from build123d import *

# Parameters (mm, degrees)
BOSS_EXTRUDE1_DEPTH = 3
SKETCH2_W           = 90
SKETCH2_H           = 44
CUT_EXTRUDE1_DEPTH  = 10
FILLET1_R           = 10
CHAMFER1_SIZE       = 15
SKETCH3_W           = 85
SKETCH3_H           = 1.6
CUT_EXTRUDE2_DEPTH  = 10
SKETCH5_W           = 3
SKETCH5_H           = 13
SKETCH5_H_2         = 8.82
SKETCH5_W_2         = 18
SKETCH5_H_3         = 3
SKETCH5_H_4         = 22.31
CUT_EXTRUDE3_DEPTH  = 10
CUT_EXTRUDE4_DEPTH  = 10
SKETCH7_R           = 10.631131443
SKETCH7_R_2         = 8.661974079
SKETCH7_R_3         = 5.563912072
SKETCH7_R_4         = 5.743787148
SKETCH7_R_5         = 6.57513677
SKETCH7_R_6         = 8.998042507
SKETCH7_R_7         = 11.788086797
SKETCH7_R_8         = 9.954868747
SKETCH7_R_9         = 6.082926802
SKETCH7_R_10        = 4.464279257
SKETCH7_R_11        = 4.037680116
SKETCH7_R_12        = 3.945902669
CUT_EXTRUDE5_DEPTH  = 10


with BuildPart() as part:
    # Sketch1 → Boss-Extrude1 (new body)
    with BuildSketch(Plane.XY):
        with BuildLine():
            Line((-45, 96.5), (45, 96.5))
            ThreePointArc((45, 96.5), (66.213203436, 87.713203436), (75, 66.5))
            Line((75, 66.5), (75, -56.5))
            ThreePointArc((75, -56.5), (63.284271247, -84.784271247), (35, -96.5))
            Line((35, -96.5), (0.5, -96.5))
            Line((0.5, -96.5), (-0.5, -96.5))
            Line((-0.5, -96.5), (-35, -96.5))
            ThreePointArc((-35, -96.5), (-63.284271247, -84.784271247), (-75, -56.5))
            Line((-75, -56.5), (-75, 66.5))
            ThreePointArc((-75, 66.5), (-66.213203436, 87.713203436), (-45, 96.5))
        make_face()
    extrude(amount=BOSS_EXTRUDE1_DEPTH)

    # Sketch2 → Cut-Extrude1 (cut)
    with BuildSketch(Plane.XY.offset(3)):
        with Locations((0, -34.5)):
            Rectangle(SKETCH2_W, SKETCH2_H)
    extrude(amount=-CUT_EXTRUDE1_DEPTH, mode=Mode.SUBTRACT)

    # Fillet1
    fillet1_edges = [part.edges().sort_by_distance(p)[0] for p in [
        (45, -56.5, 1.5),
        (-45, -56.5, 1.5),
    ]]
    fillet(fillet1_edges, radius=FILLET1_R)

    # Chamfer1
    chamfer1_edges = [part.edges().sort_by_distance(p)[0] for p in [
        (45, -12.5, 1.5),
        (-45, -12.5, 1.5),
    ]]
    chamfer(chamfer1_edges, length=CHAMFER1_SIZE)

    # Sketch3 → Cut-Extrude2 (cut)
    with BuildSketch(Plane(origin=(0, 0, 0), x_dir=(-1, 0, 0), z_dir=(0, 0, -1))):
        with Locations((0, -13.3)):
            Rectangle(SKETCH3_W, SKETCH3_H)
    extrude(amount=-CUT_EXTRUDE2_DEPTH, mode=Mode.SUBTRACT)

    # Sketch5 → Cut-Extrude3 (cut)
    with BuildSketch(Plane(origin=(0, 0, 0), x_dir=(-1, 0, 0), z_dir=(0, 0, -1))):
        with Locations((-73.5, 60)):
            Rectangle(SKETCH5_W, SKETCH5_H)
        with Locations((-40.5, 85.09)):
            Rectangle(SKETCH5_W, SKETCH5_H_2)
        with Locations((73.5, 60)):
            Rectangle(SKETCH5_W, SKETCH5_H)
        with Locations((40.5, 85.09)):
            Rectangle(SKETCH5_W, SKETCH5_H_2)
        with Locations((-49, -62.69)):
            Rectangle(SKETCH5_W_2, SKETCH5_H_3)
        with Locations((49, -62.69)):
            Rectangle(SKETCH5_W_2, SKETCH5_H_3)
        with Locations((28.5, -85.345)):
            Rectangle(SKETCH5_W, SKETCH5_H_4)
        with Locations((-28.5, -85.345)):
            Rectangle(SKETCH5_W, SKETCH5_H_4)
    extrude(amount=-CUT_EXTRUDE3_DEPTH, mode=Mode.SUBTRACT)

    # Sketch6 → Cut-Extrude4 (cut)
    with BuildSketch(Plane(origin=(0, 0, 0), x_dir=(-1, 0, 0), z_dir=(0, 0, -1))):
        with BuildLine():
            Line((-24.212655847, 72.63796754), (24.212655847, 72.63796754))
            ThreePointArc((24.212655847, 72.63796754), (58.665446775, 38.185176612), (24.212655847, 3.732385684))
            Line((24.212655847, 3.732385684), (-24.212655847, 3.732385684))
            ThreePointArc((-24.212655847, 3.732385684), (-58.665446775, 38.185176612), (-24.212655847, 72.63796754))
        make_face()
    extrude(amount=-CUT_EXTRUDE4_DEPTH, mode=Mode.SUBTRACT)

    # Sketch7 → Cut-Extrude5 (cut)
    with BuildSketch(Plane(origin=(0, 0, 0), x_dir=(-1, 0, 0), z_dir=(0, 0, -1))):
        with Locations((-56.155531371, 77.040268603)):
            Circle(SKETCH7_R)
        with Locations((-26.105041506, 84.696444365)):
            Circle(SKETCH7_R_2)
        with Locations((-63.23749395, 58.091233593)):
            Circle(SKETCH7_R_3)
        with Locations((-66.021045237, 42.587477675)):
            Circle(SKETCH7_R_4)
        with Locations((-66.021045237, 25.361082211)):
            Circle(SKETCH7_R_5)
        with Locations((-58.260979705, 4.306598866)):
            Circle(SKETCH7_R_6)
        with Locations((-60.749236828, -19.427545996)):
            Circle(SKETCH7_R_7)
        with Locations((-59.983619252, -46.60696995)):
            Circle(SKETCH7_R_8)
        with Locations((-8.495837254, 84.696444365)):
            Circle(SKETCH7_R_9)
        with Locations((-39.120540301, -6.220642806)):
            Circle(SKETCH7_R_10)
        with Locations((-26.105041506, -6.220642806)):
            Circle(SKETCH7_R_11)
        with Locations((-13.855160287, -6.220642806)):
            Circle(SKETCH7_R_12)
        with Locations((13.855160287, -6.220642806)):
            Circle(SKETCH7_R_12)
        with Locations((26.105041506, -6.220642806)):
            Circle(SKETCH7_R_11)
        with Locations((39.120540301, -6.220642806)):
            Circle(SKETCH7_R_10)
        with Locations((8.495837254, 84.696444365)):
            Circle(SKETCH7_R_9)
        with Locations((59.983619252, -46.60696995)):
            Circle(SKETCH7_R_8)
        with Locations((60.749236828, -19.427545996)):
            Circle(SKETCH7_R_7)
        with Locations((58.260979705, 4.306598866)):
            Circle(SKETCH7_R_6)
        with Locations((66.021045237, 25.361082211)):
            Circle(SKETCH7_R_5)
        with Locations((66.021045237, 42.587477675)):
            Circle(SKETCH7_R_4)
        with Locations((63.23749395, 58.091233593)):
            Circle(SKETCH7_R_3)
        with Locations((26.105041506, 84.696444365)):
            Circle(SKETCH7_R_2)
        with Locations((56.155531371, 77.040268603)):
            Circle(SKETCH7_R)
    extrude(amount=-CUT_EXTRUDE5_DEPTH, mode=Mode.SUBTRACT)


solid = part.part
Source: CAD feature listing. Evaluate the final solid. Frame: model axes, mm. A direction names the side the tool comes from. Coordinates: 2 decimals unless noted, no trailing zeros. Loops run counter-clockwise (first coordinate to the right, second up) from the corner with the lowest first, then second, coordinate; pieces in that order, holes last. Notation, with made-up numbers: (-40, -13.75) - (1, -13.75) arc R18 ccw to (1, 3.25) - close; hole circle Ø1 at (20, 64.25). An arc over 180 degrees is marked (long way). One line per item, written item: value. Start each with the question number.
1. Section C-C (x = 4.5). Return the cut outline in (y, z), and give its area (3 significant figures).
2. Section A-A (x = -53.5). Return the cut outline in (y, z), and give its area (3 significant figures).
3. Section D-D (z = 1.45). State how many separate pieces and enclosed holes the cut face has, and give its area (3 significant figures).
4. Mould query, pull axis X, two halves, no side actions, for faces 1 (the cylindrical face through (-66.573, 0.86, 1.479)), 2 (the cylindrical face through (-62.972, -85.094, 1.479)), 3 (the cylindrical face through (65.979, 87.945, 1.479)). Classes: pulls with the +X half, pulls with the -X half, needs draft (parallel to the pull), parting line crosses it, or undercut.
5. Contact query for flat-ended pins moving along their axis: P1, Ø13, axis at x = 56.16, y = 77.04, coming from the -Z side; P2, Ø0.9, axis at y = -63, z = 1, coming from the -X side; P3, Ø1.5, axis at y = 58, z = 2, coming from the -X side; P4, Ø1, axis at y = 68.5, z = 2, coming from the +X side. Output: stop coordinate, or through.
6. Set-up query: faces 4 (the flat face through (-38.4, -20.9, 1.5)), 5 (the cylindrical face through (63.594, -84.472, 1.479)). Return all of +Z, -Z, +X, -X, +Y, -Y with unobstructed straight access to the full face (end or side cutting, diameter ignored); none if empty.
7. Section B-B (y = -83). Return the cut outline in (x, z).
8. Ray query, L1, parallel to X at y = -47, z = 2.65; L2, parallel to Y at x = -68, z = 0.7; L3, parallel to X at y = 68.5, z = 1.2. Return the intervals inside material, ascending.
Verdict:
1. outline: (-96.5, 0) - (-56.5, 0) - (-56.5, 3) - (-96.5, 3) - close; (-12.5, 0) - (3.73, 0) - (3.73, 3) - (-12.5, 3) - close; (72.64, 0) - (80.11, 0) - (80.11, 3) - (72.64, 3) - close; (89.28, 0) - (96.5, 0) - (96.5, 3) - (89.28, 3) - close
1. area: 213 mm2
2. outline: (-91.96, 0) - (-64.19, 0) - (-64.19, 3) - (-91.96, 3) - close; (-61.19, 0) - (-54.16, 0) - (-54.16, 3) - (-61.19, 3) - close; (-39.05, 0) - (-28.72, 0) - (-28.72, 3) - (-39.05, 3) - close; (-10.13, 0) - (-3.33, 0) - (-3.33, 3) - (-10.13, 3) - close; (11.94, 0) - (20.04, 0) - (20.04, 3) - (11.94, 3) - close; (56.33, 0) - (66.75, 0) - (66.75, 3) - (56.33, 3) - close; (87.33, 0) - (95.27, 0) - (95.27, 3) - (87.33, 3) - close
2. area: 235 mm2
3. separate pieces: 1
3. enclosed holes: 30
3. area: 12,300 mm2
4. face 1: undercut
4. face 2: pulls with the -X half
4. face 3: pulls with the +X half
5. P1: passes through
5. P2: stops at x = -74.54
5. P3: stops at x = -72
5. P4: stops at x = 74.96
6. face 4: +Z, -Z
6. face 5: +Z, -Z, +X, -Y
7. outline: (-64.96, 0) - (-30, 0) - (-30, 3) - (-64.96, 3) - close; (-27, 0) - (27, 0) - (27, 3) - (-27, 3) - close; (30, 0) - (64.96, 0) - (64.96, 3) - (30, 3) - close
8. L1: x = -75 to -69.93, -50.04 to -44.99, 44.99 to 50.04, 69.93 to 75
8. L2: y = -79.11 to -52.51, -40.7 to -28.72, -10.13 to 19.09, 31.63 to 37.2, 47.98 to 55.21, 60.97 to 85.76
8. L3: x = -74.93 to -62.49, -49.82 to -40.58, 40.58 to 49.82, 62.49 to 74.93
